from build123d import *

# Parameters (mm, degrees)
F0_R        = 19
F1_DEPTH    = 2
F2_R        = 17.25
F3_DEPTH    = 2
F5_DEPTH    = 25
F7_DEPTH    = 6
F8_T1_DEPTH = 27
F9_R        = 2
F10_DEPTH   = 25
F11_R       = 2
F12_DEPTH   = 25
F13_R       = 2
F14_DEPTH   = 25


# Not quite as in the source:
# - a fillet or chamfer that OpenCascade refuses, or shapes differently, is made with other operations: its cross-section is extruded or revolved along the edge and cut away or added


with BuildPart() as f1:
    # F0 (on Top) → F1 (new body)
    with BuildSketch(Plane.XY):
        Circle(F0_R)
    extrude(amount=F1_DEPTH)

    # F2 (on face) → F3 (join)
    with BuildSketch(Plane.XY.offset(2)):
        Circle(F2_R)
    extrude(amount=F3_DEPTH)

    # F4 (on face) → F5 (cut)
    with BuildSketch(Plane.XY.offset(4)):
        with BuildLine():
            Line((0, 0), (8.5, 0))
            ThreePointArc((8.5, 0), (0, 8.5), (-8.5, 0))
            Line((-8.5, 0), (0, 0))
        make_face()
        with BuildLine():
            ThreePointArc((-8.5, 0), (0, -8.5), (8.5, 0))
            Line((8.5, 0), (0, 0))
            Line((0, 0), (-8.5, 0))
        make_face()
        with BuildLine():
            Line((8.5, -31.9736860693), (8.5, -15.0104130523))
            ThreePointArc((8.5, -15.0104130523), (0, -17.25), (-8.5, -15.0104130523))
            Line((-8.5, -15.0104130523), (-8.5, -31.0855284333))
            Line((-8.5, -31.0855284333), (8.5, -31.9736860693))
        make_face()
        with BuildLine():
            Line((8.5, -15.0104130523), (8.5, 0))
            ThreePointArc((8.5, 0), (0, -8.5), (-8.5, 0))
            Line((-8.5, 0), (-8.5, -15.0104130523))
            ThreePointArc((-8.5, -15.0104130523), (0, -17.25), (8.5, -15.0104130523))
        make_face()
    extrude(amount=-F5_DEPTH, mode=Mode.SUBTRACT)

    # F6 (on Top) → F7 (join)
    with BuildSketch(Plane.XY):
        with BuildLine():
            ThreePointArc((-7.75, 0), (0, 7.75), (7.75, 0))
            Line((7.75, 0), (7.75, -14))
            Line((7.75, -14), (9.75, -14))
            Line((9.75, -14), (9.75, 11))
            Line((9.75, 11), (-9.75, 11))
            Line((-9.75, 11), (-9.75, -14))
            Line((-9.75, -14), (-7.75, -14))
            Line((-7.75, -14), (-7.75, 0))
        make_face()
    extrude(amount=F7_DEPTH)

    # F8: fillet of radius 10 on 2 edges, made by hand

    # F8_s2 → F8_t1 (cut)
    with BuildSketch(Plane.XY.offset(4)):
        with BuildLine():
            ThreePointArc((9.75, 1), (6.8210678119, 8.0710678119), (-0.25, 11))
            Line((-0.25, 11), (9.75, 11))
            Line((9.75, 11), (9.75, 1))
        make_face()
        with BuildLine():
            ThreePointArc((0.25, 11), (-6.8210678119, 8.0710678119), (-9.75, 1))
            Line((-9.75, 1), (-9.75, 11))
            Line((-9.75, 11), (0.25, 11))
        make_face()
    extrude(amount=F8_T1_DEPTH, mode=Mode.SUBTRACT)

    # F9 (on face) → F10 (cut)
    with BuildSketch(Plane.XY.offset(2)):
        with Locations((14, 0)):
            Circle(F9_R)
        with BuildLine():
            ThreePointArc((-16, 0), (-14, -2), (-12, 0))
            ThreePointArc((-12, 0), (-14, 2), (-16, 0))
        make_face()
    extrude(amount=-F10_DEPTH, mode=Mode.SUBTRACT)

    # F11 (on face) → F12 (cut)
    with BuildSketch(Plane(origin=(0, 0, 2), x_dir=(1, 0, 0), z_dir=(0, 0, -1))):
        with Locations((-14, 0)):
            Circle(F11_R)
    extrude(amount=-F12_DEPTH, mode=Mode.SUBTRACT)

    # F13 (on face) → F14 (cut)
    with BuildSketch(Plane(origin=(0, 0, 2), x_dir=(1, 0, 0), z_dir=(0, 0, -1))):
        with Locations((14, 0)):
            Circle(F13_R)
    extrude(amount=-F14_DEPTH, mode=Mode.SUBTRACT)


solid = f1.part
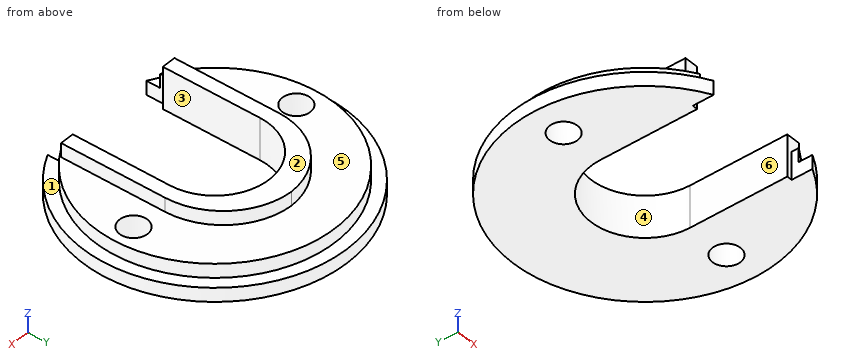
Design review of the part built by this model. Coordinates are the model's own, in mm. Face numbers are marked on the shaded views. A direction names the side the tool comes from. Give positions to 0.01 mm unless a question says otherwise; leave off trailing zeros. Loops run counter-clockwise (first coordinate to the right, second up) from the corner with the lowest first, then second, coordinate; pieces in that order, holes last. Notation, with made-up numbers: M 13.5,37.5 L 38.5,37.5 A32 ccw 38.5,74.5 Z; hole C 7,42.25 d7. An arc over 180 degrees is marked long. Write item = value, one per line.
Q1. We need section B-B (z = 0.9). Give the boundary of the cut face in (x, y).
Output values:
outline = M -8.5,-16.99 L -8.5,-14 L -7.75,-14 L -7.75,0 A7.75 cw 7.75,0 L 7.75,-14 L 8.5,-14 L 8.5,-16.99 A19 ccw long Z; hole C -14,0 d4; hole C 14,0 d4
Q2. Draft analysis for pull direction X (two halves, no side actions). For the marked faces 4, 5 and 6, state which applies: +X half, -X half, draft (parallel to the pull), parting line (faces both ways), or undercut.
Output values:
face_4 = undercut
face_5 = draft
face_6 = undercut
Q3. Insertion check: pin 1 (1.5 mm diameter, centred on x = 8, z = 4, fed in from -Y); pin 2 (0.9 mm diameter, centred on y = -15, z = 2, fed in from +X); pin 3 (1.8 mm diameter, centred on y = -6, z = 2.5, fed in from +X). Each pin has a flat end and moves straight along its axis. Give the tip position at first contact, or say it passes through.
Output values:
pin_1 = -15.01
pin_2 = 12.22
pin_3 = 18.26
Q4. We need section D-D (z = 3.4). Give the boundary of the cut face in (x, y).
Output values:
outline = M -8.5,-15.01 L -8.5,-14 L -7.75,-14 L -7.75,0 A7.75 cw 7.75,0 L 7.75,-14 L 8.5,-14 L 8.5,-15.01 A17.25 ccw long Z; hole C -14,0 d4; hole C 14,0 d4
Q5. For the marked faces 1, 2 and 3, list the 3-axis set-ups (+Z, -Z, +X, -X, +Y, -Y) from which the entire face can be reached by the end or side of a thin tool; tool diameter is ignored.
Output values:
face_1 = +Z
face_2 = +Z, +X, -X, +Y, -Y
face_3 = +Z, -Z, -Y
Q6. We need section C-C (y = 14). Give the boundary of the cut face in (x, z).
Output values:
outline = M -12.85,0 L 12.85,0 L 12.85,2 L 10.08,2 L 10.08,4 L -10.08,4 L -10.08,2 L -12.85,2 Z
Q7. To check wall thickness, follow line 1 (X direction, y = -10.5, z = 4.4); line 2 (Z direction, x = -10.5, y = 1); line 3 (X direction, y = -7.5, z = 2.3). State the ranges of each line that lie inside material, in increasing order. Write a range as [from, to].
Output values:
line_1 = [-9.75, -7.75], [7.75, 9.75]
line_2 = [0, 4]
line_3 = [-15.53, -7.75], [7.75, 15.53]
Q8. We need section A-A (x = -14.5). Give the boundary of the cut face in (y, z).
Output values:
outline = M -12.28,0 L -1.94,0 L -1.94,4 L -9.34,4 L -9.34,2 L -12.28,2 Z; M 1.94,0 L 12.28,0 L 12.28,2 L 9.34,2 L 9.34,4 L 1.94,4 Z
